from build123d import *

# Parameters (mm, degrees)
SKETCH1_W           = 40
SKETCH1_H           = 50
SKETCH1_R           = 2.5
BOSS_EXTRUDE1_DEPTH = 6.35
FILLET1_R           = 15


with BuildPart() as part:
    # Sketch1 → Boss-Extrude1 (new body)
    with BuildSketch(Plane(origin=(0, 0, 0), x_dir=(1, 0, 0), z_dir=(0, 1, 0))):
        with Locations((1.322957198, 0.214007782)):
            Rectangle(SKETCH1_W, SKETCH1_H)
        with Locations(Location((1.322957198, -2.33463035, 0), (0, 0, 270))):
            Circle(SKETCH1_R, mode=Mode.SUBTRACT)
    extrude(amount=BOSS_EXTRUDE1_DEPTH)

    # Fillet1
    fillet1_edges = [part.edges().sort_by_distance(p)[0] for p in [
        (21.322957198, 3.175, 24.785992218),
        (-18.677042802, 3.175, 24.785992218),
    ]]
    fillet(fillet1_edges, radius=FILLET1_R)


solid = part.part
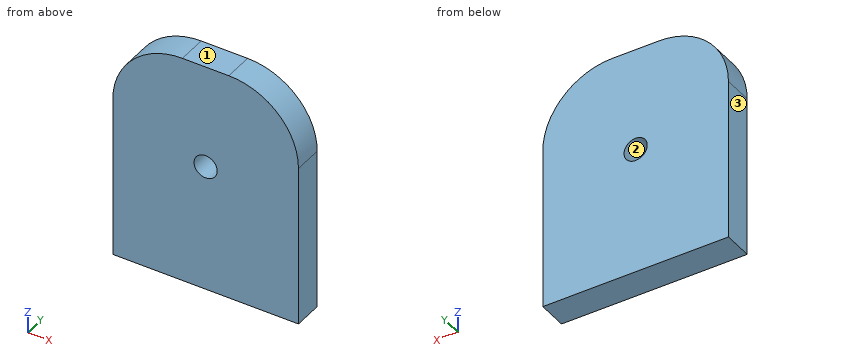
Build history of the part. All positions in model axes, mm. Face numbers are marked on the shaded views. Round coordinates to 2 decimals unless told otherwise and drop trailing zeros. Write each loop counter-clockwise with the first axis right and the second up, starting at its lowest first coordinate (ties: lowest second). Pieces come first, ordered by that corner, then holes. Notation, with made-up numbers: (45.5, 23.25) - (64.5, 23.25) arc R13 ccw to (64.5, 48.25) - close; hole circle Ø1 at (22.25, -27). An arc over 180 degrees is marked (long way). One line per question, with ' | ' between items.
1. Mould opens along Z. For the marked faces 1, 2 and 3 say: released by +Z, released by -Z, zero draft, split by the parting line, or undercut.
Results are:
face 1: released by +Z | face 2: undercut | face 3: zero draft
2. Band-saw the part on D-D, the plane x = -8.5. Write the cut outline in (y, z).
Results are:
outline: (0, -25.21) - (6.35, -25.21) - (6.35, 23.99) - (0, 23.99) - close
3. Drop flat-ended pins along their axis: pin 1 Ø1.5 at (y, z) = (5.5, 19) entering from +X; pin 2 Ø5 at (x, z) = (1, 1) entering from +Y. Give the stop position or say it passes through.
Results are:
pin 1: x = 18.71 | pin 2: y = 6.35
4. Band-saw the part on A-A, the plane z = 4. Write the cut outline in (x, y), and give its area (3 significant figures).
Results are:
outline: (-18.68, 0) - (-0.54, 0) - (-0.54, 6.35) - (-18.68, 6.35) - close; (3.19, 0) - (21.32, 0) - (21.32, 6.35) - (3.19, 6.35) - close | area: 230 mm^2
5. Band-saw the part on B-B, the plane x = 3. Write the cut outline in (y, z).
Results are:
outline: (0, -25.21) - (6.35, -25.21) - (6.35, 0.48) - (0, 0.48) - close; (0, 4.19) - (6.35, 4.19) - (6.35, 24.79) - (0, 24.79) - close
6. Band-saw the part on C-C, the plane y = 4.5. Write the cut outline in (x, z).
Results are:
outline: (-18.68, -25.21) - (21.32, -25.21) - (21.32, 9.79) arc R15 ccw to (6.32, 24.79) - (-3.68, 24.79) arc R15 ccw to (-18.68, 9.79) - close; hole circle Ø5 at (1.32, 2.33)
7. Drill centre lines: line 1 along Z through (x, y) = (1.5, 0.5); line 2 along X through (y, z) = (3.75, 4); line 3 along Z through (x, y) = (0.5, 6). Where is each one in solid material? Low to high. Write a range as from..to.
Results are:
line 1: -25.21..-0.16, 4.83..24.79 | line 2: -18.68..-0.54, 3.19..21.32 | line 3: -25.21..-0.03, 4.7..24.79
